The listing builds one solid part. Answer for the finished solid, in the listing's coordinates (mm). A direction names the side the tool comes from. Round coordinates to 2 decimals unless told otherwise and drop trailing zeros. Order: outer loops, then holes, each group sorted by start corner. A loop starts at its lowest first (then second) coordinate and runs counter-clockwise, first axis right, second up. Notation, with made-up numbers: (58, 68) -> (112, 68) arc R15 ccw to (112, 74) -> close; hole circle Ø6 at (61.5, -20.5). An arc over 180 degrees is marked (long way). Answer in a Markdown table with one row per item. Add a question column.
```python
from build123d import *

# Parameters (mm, degrees)
FEMALE_M3_HEX_STANDOFF_AF5_SKETCH_R = 1.51
FEMALE_M3_HEX_STANDOFF_AF5_DEPTH    = 16.5
STUD_ROOT_SKETCH_R                  = 1.85
STUD_ROOT_DEPTH                     = 0.45
MALE_M3_STUD_ENVELOPE_START         = -2
MALE_M3_STUD_ENVELOPE_SKETCH_R      = 1.5
MALE_M3_STUD_ENVELOPE_DEPTH         = 2


with BuildPart() as part:
    # Female_M3_hex_standoff_AF5_Sketch → Female_M3_hex_standoff_AF5 (new body)
    with BuildSketch(Plane.XY):
        Polygon((2.886751346, 0), (1.443375673, 2.5), (-1.443375673, 2.5), (-2.886751346, 0), (-1.443375673, -2.5), (1.443375673, -2.5), align=None)
        Circle(FEMALE_M3_HEX_STANDOFF_AF5_SKETCH_R, mode=Mode.SUBTRACT)
    extrude(amount=FEMALE_M3_HEX_STANDOFF_AF5_DEPTH)

    # Stud_root_Sketch → Stud_root (add)
    with BuildSketch(Plane.XY):
        Circle(STUD_ROOT_SKETCH_R)
    extrude(amount=STUD_ROOT_DEPTH)

    # Male_M3_stud_envelope_Sketch → Male_M3_stud_envelope (add)
    with BuildSketch(Plane.XY.offset(MALE_M3_STUD_ENVELOPE_START)):
        Circle(MALE_M3_STUD_ENVELOPE_SKETCH_R)
    extrude(amount=MALE_M3_STUD_ENVELOPE_DEPTH)


solid = part.part
```
1. For faces 1 (the flat face through (0, 0, -2)), 2 (the cylindrical face through (-1.5, 0.07, -1.01)), determine the directions among +Z, -Z, +X, -X, +Y, -Y from which every point of the face is accessible in a straight line to the end or side of a thin tool.
2. Straight lines are drawn through the part: line 1 along Y through (x, z) = (0, 4); line 2 along Z through (x, y) = (-2.4, 0.75); line 3 along X through (y, z) = (-0.5, 4.25). For each, find the intervals that lie inside material, in ascending order.
3. This flat-tipped pin is pushed along its axis until it touches: pin 1 (1 mm diameter, centred on y = 2, z = 11.5, fed in from -X). Where does it stop, or does it pass through?
4. The part is cut by section A-A (z = 10.25). Give the vertices of the cut face in (x, y), then the cut area to 3 significant figures.
5. The part is cut by section D-D (y = 1.95). Give the vertices of the cut face in (x, z), then the cut area to 3 significant figures.
6. The mould has two halves that part along X. Classify faces 3 (the flat face through (-2.155, 1.267, 8.134)), 4 (the cylindrical face through (-0.197, 1.497, 8.363)), 5 (the flat face through (0, 0, 0.45)), 6 (the flat face through (2.155, -1.267, 8.134)): released by +X, released by -X, zero draft, split by the parting line, or undercut.
7. The part is cut by section B-B (x = 0). Give the vertices of the cut face in (y, z).
8. The part is cut by section C-C (y = 0.75). Give the vertices of the cut face in (x, z).
Report:
| question | item | result |
|---|---|---|
| 1 | face 1 | -Z, +X, -X, +Y, -Y |
| 1 | face 2 | -Z |
| 2 | line 1 | y = -2.5 to -1.51, 1.51 to 2.5 |
| 2 | line 2 | z = 0 to 16.5 |
| 2 | line 3 | x = -2.6 to -1.42, 1.42 to 2.6 |
| 3 | pin 1 | stops at x = -2.02 |
| 4 | outline | (-2.89, 0) -> (-1.44, -2.5) -> (1.44, -2.5) -> (2.89, 0) -> (1.44, 2.5) -> (-1.44, 2.5) -> close; hole circle Ø3.02 at (0, 0) |
| 4 | area | 14.5 mm^2 |
| 5 | outline | (-1.76, 0) -> (1.76, 0) -> (1.76, 16.5) -> (-1.76, 16.5) -> close |
| 5 | area | 58.1 mm^2 |
| 6 | face 3 | released by -X |
| 6 | face 4 | undercut |
| 6 | face 5 | undercut |
| 6 | face 6 | released by +X |
| 7 | outline | (-2.5, 0) -> (-1.5, 0) -> (-1.5, -2) -> (1.5, -2) -> (1.5, 0) -> (2.5, 0) -> (2.5, 16.5) -> (1.51, 16.5) -> (1.51, 0.45) -> (-1.51, 0.45) -> (-1.51, 16.5) -> (-2.5, 16.5) -> close |
| 8 | outline | (-2.45, 0) -> (-1.3, 0) -> (-1.3, -2) -> (1.3, -2) -> (1.3, 0) -> (2.45, 0) -> (2.45, 16.5) -> (1.31, 16.5) -> (1.31, 0.45) -> (-1.31, 0.45) -> (-1.31, 16.5) -> (-2.45, 16.5) -> close |
